Check sheet for the drawn part. Datum: minimum x, y, z corner. Units: mm. A direction names the side the tool comes from. Give positions to 0.01 mm unless a question says otherwise; leave off trailing zeros. Loops run counter-clockwise (first coordinate to the right, second up) from the corner with the lowest first, then second, coordinate; pieces in that order, holes last.
1. Cross-section at C-C, the plane x = 0.3. Record the cut outline in (y, z), plus the area to 3 significant figures.
2. Cross-section at B-B, the plane z = 2.5. Record the cut outline in (x, y), plus the area to 3 significant figures.
3. Cross-section at A-A, the plane x = 2.5. Record the cut outline in (y, z).
4. Tool access check on the marked faces 1, 2 and 3. Record the directions out of +Z, -Z, +X, -X, +Y, -Y that give a thin tool (end or side, any length) a straight path to the whole face; none if there is none.
5. Material ranges on L1, parallel to Z at x = 3, y = 15.25; L2, parallel to Y at x = 1.1, z = 3.5; L3, parallel to Y at x = 3.6, z = 1, recorded low to high.
6. Go/stop test with flat-tipped pins: pin 1 Ø1.6 at (x, z) = (1.5, 8.5) entering from +Y; pin 2 Ø1.6 at (x, y) = (2, 4.5) entering from +Z; pin 3 Ø2.5 at (y, z) = (3, 6.5) entering from +X; pin 4 Ø3 at (x, z) = (3.5, 4.5) entering from +Y. Record where each tip stops, or that it passes through.
7. Cross-section at D-D, the plane y = 4.5. Record the cut outline in (x, z).
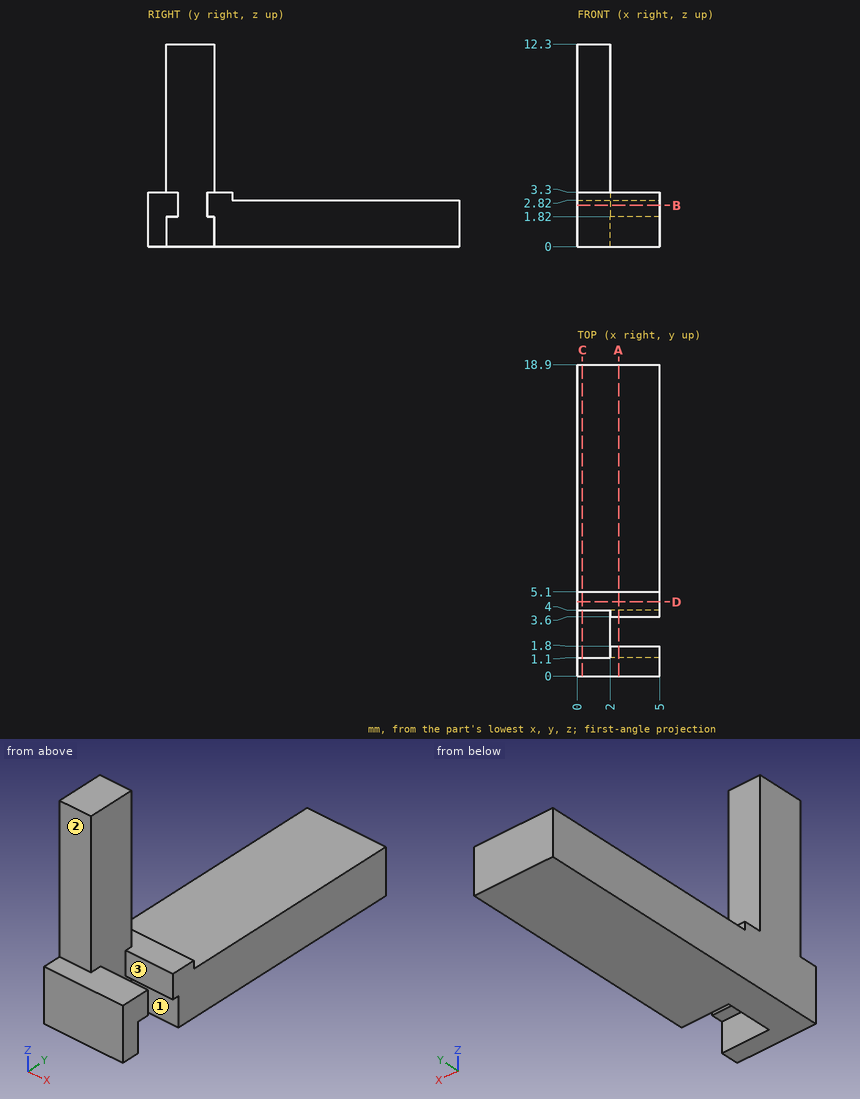
Result:
1. outline: (0, 0) - (18.9, 0) - (18.9, 2.82) - (5.1, 2.82) - (5.1, 3.3) - (4, 3.3) - (4, 12.3) - (1.1, 12.3) - (1.1, 3.3) - (0, 3.3) - close
1. area: 81.8 mm2
2. outline: (0, 0) - (5, 0) - (5, 1.8) - (2, 1.8) - (2, 3.6) - (5, 3.6) - (5, 18.9) - (0, 18.9) - close
2. area: 89.1 mm2
3. outline: (0, 0) - (1.1, 0) - (1.1, 1.82) - (1.8, 1.82) - (1.8, 3.3) - (0, 3.3) - close; (3.6, 1.82) - (4, 1.82) - (4, 0) - (18.9, 0) - (18.9, 2.82) - (5.1, 2.82) - (5.1, 3.3) - (3.6, 3.3) - close
4. face 1: -Z, +X
4. face 2: +Z, +X, -X, -Y
4. face 3: +Z, -Z, +X
5. L1: z = 0 to 2.82
5. L2: y = 1.1 to 4
5. L3: y = 0 to 1.1, 4 to 18.9
6. pin 1: stops at y = 4
6. pin 2: stops at z = 12.3
6. pin 3: stops at x = 2
6. pin 4: stops at y = 5.1
7. outline: (0, 0) - (5, 0) - (5, 3.3) - (0, 3.3) - close
